Here's how the part is built. I have some questions about the finished solid (model axes, mm). Face numbers are marked on the shaded views. A direction names the side the tool comes from. Coordinates: 2 decimals unless noted, no trailing zeros. Order: outer loops, then holes, each group sorted by start corner. A loop starts at its lowest first (then second) coordinate and runs counter-clockwise, first axis right, second up. Notation, with made-up numbers: (64, 67.25) - (76, 67.25) arc R4 cw to (76, 73.25) - close; hole circle Ø1 at (6, 70.5). An arc over 180 degrees is marked (long way). Answer in a Markdown table with one row per item. Add a question column.
Item 1: Will these pins go through, and if not, where does the flat tip stop? pin 1 Ø7 at (x, y) = (15.5, 9) entering from -Z; pin 2 Ø10 at (x, y) = (33, 11.5) entering from -Z; pin 3 Ø6 at (x, y) = (-0.5, 4.5) entering from -Z; pin 4 Ø5 at (x, z) = (11.5, 3) entering from -Y.
Item 2: I want a section at A-A (x = 37). Please give me the cut outline in (y, z), plus the area to 3 significant figures.
Item 3: On a 3-axis mill with a long thin cutter (end or side, diameter ignored), from which of +Z, -Z, +X, -X, +Y, -Y can I reach the whole of each face in a straight line? I mean the marked faces 5, 6 and 7. Say none if no direction works.
Item 4: If I drill on line 1 along X through (y, z) = (11.5, 10.5); line 2 along X through (y, z) = (8.75, 7.75); line 3 along X through (y, z) = (7, 10.2), over which ranges is the centre line in solid material (lowest first)? Write a range as from..to.
Item 5: Thinking about a two-plate mould opening in X: for the marked faces 1, 2, 3 and 4, which applies, +X half, -X half, draft (parallel to the pull), parting line (faces both ways), or undercut?
Autodesk Inventor part; units mm, degrees
ref_plane "YZ Plane" through (0, 0, 0) normal (1, 0, 0) x (0, 1, 0)
ref_plane "XZ Plane" through (0, 0, 0) normal (0, 1, 0) x (-1, 0, 0)
ref_plane "XY Plane" through (0, 0, 0) normal (0, 0, 1) x (1, 0, 0)
sketch "Sketch1" plane through (0, 0, 0) normal (0, 0, 1) x (1, 0, 0)
  line L0 (45, 0) -> (-6.5, 0)
  line L1 (-6.5, 0) -> (-6.5, 25)
  line L2 (45, 25) -> (-6.5, 25)
  line L3 (45, 0) -> (45, 25)
  circle A0 centre (12.8053, 7) radius 1.25
  circle A1 centre (20.8333, 12.9625) radius 1.25
  circle A2 centre (34, 9) radius 3
extrude "Bryla" add sketch "Sketch1" along normal blind 11 contours L0 L1 L2 L3 | A0 | A1 | A2
sketch "Sketch3" plane through (0, 0, 0) normal (0, 0, -1) x (-1, 0, 0)
  circle A0 centre (-6, 12.5) radius 3.5
  circle A1 centre (-12.8053, 7) radius 7
  circle A2 centre (-20.8333, 12.9625) radius 8.25
  circle A3 centre (-34, 9) radius 11
  circle A4 centre (-34, 9) radius 4.05
  circle A5 centre (-34, 9) radius 6.1
  line L0 (-6, 12.5) -> (-12.8053, 7) construction
  line L1 (-12.8053, 7) -> (-20.8333, 12.9625) construction
  line L2 (-20.8333, 12.9625) -> (-34, 9) construction
  line L3 (-11.3429, 19.1109) -> (-0.6571, 5.8891) construction
  circle A6 centre (-0.6571, 5.8891) radius 1.7
  circle A7 centre (-11.3429, 19.1109) radius 1.7
  circle A8 centre (-11.3429, 19.1109) radius 2.8
  circle A9 centre (-0.6571, 5.8891) radius 2.8
  line L4 (6.5, 25) -> (6.5, 0) construction
  line L5 (6.5, 0) -> (-45, 0) construction
  line L6 (-45, 0) -> (-45, 25) construction
  line L7 (-34, 20) -> (-45, 20)
  line L8 (-45, 20) -> (-45, 0)
  line L9 (6.5, 0) -> (-45, 0)
  line L10 (-40.3246, 0) -> (-45, 0)
  line L11 (-27.6754, 0) -> (-23, 0)
  line L12 (-23, 0) -> (-23, 9)
  line L13 (-19.8053, 7) -> (-19.8053, 0)
  line L14 (-5.8053, 7) -> (-5.8053, 0)
  line L15 (-23, 0) -> (-19.8053, 0)
  line L16 (-29.0833, 12.9625) -> (-29.0833, 0)
  line L17 (-29.0833, 0) -> (-27.6754, 0)
  point P0 (-27.9066, 8.7162)
  point P1 (-29.0753, 12.5997)
  point P2 (-19.4597, 4.8276)
  point P3 (-22.8938, 18.8508)
  point P4 (-23.6713, 5.216)
  point P5 (-25.7685, 19.5736)
  point P6 (-12.819, 14.9204)
  point P7 (-27.4753, 17.856)
  point P8 (-20.5208, 12.676)
  point P9 (-12.6486, 13.9982)
  point P10 (-18.4098, 11.1941)
  point P11 (-8.5508, 12.5587)
  point P12 (-1.1315, 7.6691)
  point P13 (-9.5, 12.5)
  point P14 (-2.6315, 11.5495)
  point P15 (-9.4412, 13.1386)
  point P16 (-6.1553, 9.4162)
  point P17 (-8.5736, 18.697)
  point P18 (-9.3, 21.0258)
  point P19 (-6.0975, 9.0014)
  point P20 (-27.6754, 0)
  point P21 (-12.8053, 0)
  point P22 (-19.8053, 4.7768)
  point P23 (-23, 5.0021)
  dimension "d20" = 7
  dimension "d21" = 14
  dimension "d22" = 16.5
  dimension "d23" = 22
  dimension "d24" = 12.2
  dimension "d25" = 8.1
  dimension "d26" = 8.75
  dimension "d27" = 10
  dimension "d28" = 13.75
  dimension "d59" = 5.6
  dimension "d60" = 3.4
  dimension "d61" = 17
  dimension "d65" = 12.5
  dimension "d66" = 12.5
  dimension "d68" = 11
  dimension "d69" = 9
extrude "Przelot" cut sketch "Sketch3" against normal through all contours A0 A1 | A1 A0 | A4 | A6 | A7
extrude "kolo3" cut sketch "Sketch3" against normal blind 3.5 contours A1 A0 | A3 A2 A5 | A2 L16 A5 L9 A3 | L13 L9 L12 A2 | A2 A5 L16 | L12 A2 A3 | A3 L8 L7 | L12 L9 A3 A2 | A5 A2 | A2 A5 L16 | L16 A5 | A3 L9 L16 A5 A2 | A3 L9 L8 | A3 L9 | A4 picked at (-7.468, 10.5481)
extrude "kolo1" cut sketch "Sketch3" against normal blind 9.3 contours A0 A1 | A1 A0 | A0 A1 A2 | A2 A1 | L14 L9 A1 | A1 A2 L13 | L9 L13 A2 A1
extrude "kolo2" cut sketch "Sketch3" against normal blind 5.7 contours A2 A1 | A1 L13 A2 L12 A3 | A1 A2 L13 | A3 A2 A5 | L12 A2 A3 | A5 A2
hole "osieMale" at (20.8333, 12.9625, 0) at (12.8053, 7, 0) direction (0, 0, 1) diameter 2.5 end through all
extrude "kolnierzLozyska" cut sketch "Sketch3" against normal blind 1 from surface at -3.5 contours A2 A5 L16 | L16 A5 picked at (-28.8319, 8.8586)
extrude "lbySrob" cut sketch "Sketch3" against normal up to surface (9.3 mm away) contours A6 | A7 | A8 | A9
sketch "Sketch5" plane through (-6.5, 0, 11) normal (0, -1, 0) x (1, 0, 0)
  line L0 (0, -11) -> (0, 0) construction
  point P0 (6.5, -11)
  point P1 (3, -5.5)
  point P2 (0, -5.5)
  dimension "d71" = 3
hole "Hole3" at (-3.5, 0, 5.5) direction (0, 1, 0) diameter 2.459 depth 6 tip angle 118
fillet "Fillet1" radius 7 1 edges at (45, 0, 7.25)
properties part number "MocowaniePrzekladni_CPY_3DPrint"
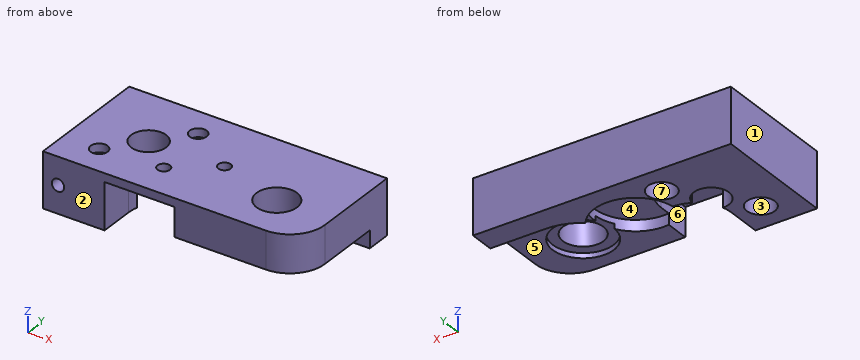
Values follow:
| question | item | result |
|---|---|---|
| 1 | pin 1 | stops at z = 9.3 |
| 1 | pin 2 | stops at z = 3.5 |
| 1 | pin 3 | stops at z = 0 |
| 1 | pin 4 | stops at y = 13.14 |
| 2 | outline | (0, 3.5) - (3.69, 3.5) - (3.69, 4.5) - (6.28, 4.5) - (6.28, 11) - (0, 11) - close; (11.72, 4.5) - (14.31, 4.5) - (14.31, 3.5) - (20, 3.5) - (20, 0) - (25, 0) - (25, 11) - (11.72, 11) - close |
| 2 | area | 159 mm^2 |
| 3 | face 5 | -Z, +X, -Y |
| 3 | face 6 | -Z, -Y |
| 3 | face 7 | -Z |
| 4 | line 1 | x = -6.5..2.65, 9.35..30.81, 37.19..45 |
| 4 | line 2 | x = -6.5..6.03, 19.58..29.96, 38.04..45 |
| 4 | line 3 | x = -6.5..-0.63, 1.94..11.56, 14.06..30.48, 37.52..45 |
| 5 | face 1 | -X half |
| 5 | face 2 | draft |
| 5 | face 3 | undercut |
| 5 | face 4 | undercut |
